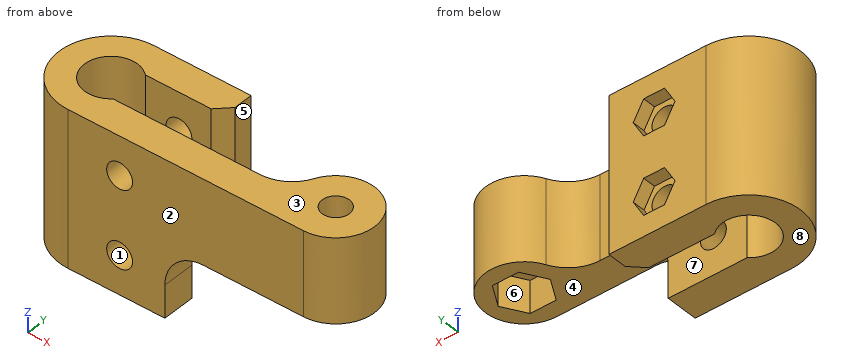
```python
from build123d import *

# Parameters (mm, degrees)
SKETCH1_R           = 2.1
BOSS_EXTRUDE1_DEPTH = 24
SKETCH2_R           = 2
CUT_EXTRUDE1_DEPTH  = 17
CUT_EXTRUDE2_DEPTH  = 2
CUT_EXTRUDE3_DEPTH  = 5
CHAMFER1_SIZE       = 2


with BuildPart() as part:
    # Sketch1 → Boss-Extrude1 (new body)
    with BuildSketch(Plane.XY):
        with BuildLine():
            Line((2.794637722, 3), (15, 3))
            Line((15, 3), (15, 8))
            Line((15, 8), (0, 8))
            ThreePointArc((0, 8), (-8, 0), (0, -8))
            Line((0, -8), (36.445164288, -8))
            ThreePointArc((36.445164288, -8), (41.494916757, 1.240370349), (30.990808231, 0.5))
            ThreePointArc((30.990808231, 0.5), (28.776822523, -2.049752469), (25.536452174, -3))
            Line((25.536452174, -3), (2.794637722, -3))
            ThreePointArc((2.794637722, -3), (-4.1, 0), (2.794637722, 3))
        make_face()
        with Locations((36.445164288, -2)):
            Circle(SKETCH1_R, mode=Mode.SUBTRACT)
    extrude(amount=BOSS_EXTRUDE1_DEPTH)

    # Sketch2 → Cut-Extrude1 (cut, through all)
    with BuildSketch(Plane.XZ.offset(8)):
        with Locations((8, 18)):
            Circle(SKETCH2_R)
        with Locations((8, 6)):
            Circle(SKETCH2_R)
        with BuildLine():
            Line((15, 5), (15, 0))
            Line((15, 0), (45.871149595, 0))
            Line((45.871149595, 0), (45.871149595, 11))
            Line((45.871149595, 11), (21, 11))
            ThreePointArc((21, 11), (16.757359313, 9.242640687), (15, 5))
        make_face()
    extrude(amount=-CUT_EXTRUDE1_DEPTH, mode=Mode.SUBTRACT)

    # Sketch3 → Cut-Extrude2 (cut)
    with BuildSketch(Plane(origin=(0, 8, 0), x_dir=(-1, 0, 0), z_dir=(0, 1, 0))):
        Polygon((-9.616580754, 8.8), (-11.233161507, 6), (-9.616580754, 3.2), (-6.383419246, 3.2), (-4.766838493, 6), (-6.383419246, 8.8), align=None)
        Polygon((-9.616580754, 20.8), (-11.233161507, 18), (-9.616580754, 15.2), (-6.383419246, 15.2), (-4.766838493, 18), (-6.383419246, 20.8), align=None)
    extrude(amount=-CUT_EXTRUDE2_DEPTH, mode=Mode.SUBTRACT)

    # Sketch4 → Cut-Extrude3 (cut)
    with BuildSketch(Plane(origin=(0, 0, 11), x_dir=(-1, 0, 0), z_dir=(0, 0, -1))):
        Polygon((-34.424438346, 1.5), (-38.46589023, 1.5), (-40.486616173, -2), (-38.46589023, -5.5), (-34.424438346, -5.5), (-32.403712404, -2), align=None)
    extrude(amount=-CUT_EXTRUDE3_DEPTH, mode=Mode.SUBTRACT)

    # Chamfer1
    chamfer1_edges = [part.edges().sort_by_distance(p)[0] for p in [
        (15, 3, 12),
    ]]
    chamfer(chamfer1_edges, length=CHAMFER1_SIZE)


solid = part.part
```
CAD build for the part. Positions are in the model's coordinates, mm. Face numbers are marked on the shaded views. A direction names the side the tool comes from. Coordinates: 2 decimals unless noted, no trailing zeros. Loops run counter-clockwise (first coordinate to the right, second up) from the corner with the lowest first, then second, coordinate; pieces in that order, holes last. Notation, with made-up numbers: (64, -5) - (90, -5) arc R19 cw to (90, 17) - close; hole circle Ø1 at (-10.5, 20). An arc over 180 degrees is marked (long way). Use CSV: the item, a comma, the result in double quotes. Start each with the question number.
Q1. Cut at C-C, the plane y = 2. List the corners of the cut face in (x, z).
Q2. Cut at B-B, the plane x = 8. State how many separate pieces and enclosed holes the cut face has, then the cut area to 3 significant figures.
Q3. Two-plate mould, pull along Z, no slides. Class the marked faces 1, 2 and 3: +Z half, -Z half, draft (parallel to the pull), parting line (faces both ways), or undercut.
Q4. 3-axis set-ups, long thin cutter, end or side, ignore diameter. For the marked faces 4, 5, 6, 7 and 8: which of +Z, -Z, +X, -X, +Y, -Y reach the whole face in a straight line?
Q5. Probe probe 1 along Z at (x, y) = (8, -4.85); probe 2 along Z at (x, y) = (8.5, -5.25); probe 3 along X at (y, z) = (-2, 18.5). List the from-to ranges inside material, lowest first. Write a range as from..to.
Q6. Drop flat-ended pins along their axis: P1, Ø5, axis at x = 0, y = 0, coming from the -Z side; P2, Ø1.5, axis at y = -3.5, z = 17.5, coming from the -X side; P3, Ø7.5, axis at x = 35.5, y = -2, coming from the -Z side; P4, Ø4.5, axis at x = 8, z = 17.5, coming from the +Y side. Give the stop position or say it passes through.
Q7. Cut at D-D, the plane z = 19.25. List the corners of the cut face in (x, y).
Q8. Cut at A-A, the plane z = 14. List the corners of the cut face in (x, y), then the cut area to 3 significant figures.
Here are the results:
1,outline,"(-7.75, 0) - (-3.58, 0) - (-3.58, 24) - (-7.75, 24) - close; (31.97, 11) - (40.92, 11) - (40.92, 24) - (31.97, 24) - close"
2,separate pieces,"6"
2,enclosed holes,"0"
2,area,"154 mm2"
3,face 1,"undercut"
3,face 2,"draft"
3,face 3,"+Z half"
4,face 4,"-Z, +X, +Y, -Y"
4,face 5,"+Z, -Z, +X, +Y"
4,face 6,"-Z"
4,face 7,"+Z, -Z"
4,face 8,"-Z, +X, -X, +Y, -Y"
5,probe 1,"0..4, 8..16, 20..24"
5,probe 2,"0..4.06, 7.94..16.06, 19.94..24"
5,probe 3,"-7.75..-3.58, 28.85..34.35, 38.55..42.45"
6,P1,"through"
6,P2,"x = -7.51"
6,P3,"z = 11"
6,P4,"y = 6"
7,outline,"(0, -8) - (6.44, -8) - (6.44, -3) - (2.79, -3) arc R4.1 cw (long way) to (2.79, 3) - (6.44, 3) - (6.44, 6) - (5.49, 6) - (5.49, 8) - (0, 8) arc R8 ccw to start; (9.56, -8) - (36.45, -8) arc R6 ccw (long way) to (30.99, 0.5) arc R6 cw to (25.54, -3) - (9.56, -3) - close; (9.56, 3) - (13, 3) - (15, 5) - (15, 8) - (10.51, 8) - (10.51, 6) - (9.56, 6) - close; hole circle Ø4.2 at (36.45, -2)"
8,outline,"(0, -8) - (36.45, -8) arc R6 ccw (long way) to (30.99, 0.5) arc R6 cw to (25.54, -3) - (2.79, -3) arc R4.1 cw (long way) to (2.79, 3) - (13, 3) - (15, 5) - (15, 8) - (0, 8) arc R8 ccw to start; hole (32.4, -2) - (34.42, -5.5) - (38.47, -5.5) - (40.49, -2) - (38.47, 1.5) - (34.42, 1.5) - close"
8,area,"377 mm2"
